Part model, mm, in its own coordinate system. A direction names the side the tool comes from. Coordinates: 2 decimals unless noted, no trailing zeros. Write each loop counter-clockwise with the first axis right and the second up, starting at its lowest first coordinate (ties: lowest second). Pieces come first, ordered by that corner, then holes. Notation, with made-up numbers: (-1.75, 51.25) - (29.25, 51.25) arc R18 cw to (29.25, 76.25) - close; hole circle Ø11 at (86, 62.25). An arc over 180 degrees is marked (long way). Use a Markdown table: item, result.
```python
from build123d import *

# Parameters (mm, degrees)
F3_DEPTH = 25.4
F4_R     = 3.175
F5_DEPTH = 18.3706396773


with BuildPart() as f1:
    # F0 (on Front) → F1 (revolve)
    with BuildSketch(Plane.XZ):
        with BuildLine():
            Line((6.35, 12.0196396773), (-120.65, 12.0196396773))
            Line((-120.65, 12.0196396773), (-120.65, 10.49467489))
            ThreePointArc((-120.65, 10.49467489), (-116.3146984161, 6.0237057619), (-114.733757664, 0))
            Line((-114.733757664, 0), (6.35, 0))
            Line((6.35, 0), (6.35, 12.0196396773))
        make_face()
    revolve(axis=Axis((-54.191878832, 0, 0), (-1, 0, 0)))

    # F2 (on face) → F3 (cut)
    with BuildSketch(Plane.YZ.offset(6.35)):
        with BuildLine():
            Line((-6.35, -10.2053533977), (-6.35, 10.2053533977))
            ThreePointArc((-6.35, 10.2053533977), (-12.0196396773, 0), (-6.35, -10.2053533977))
        make_face()
        with BuildLine():
            ThreePointArc((12.0196396773, 0), (10.5070559607, 5.8372521798), (6.35, 10.2053533977))
            Line((6.35, 10.2053533977), (6.35, -10.2053533977))
            ThreePointArc((6.35, -10.2053533977), (10.5070559607, -5.8372521798), (12.0196396773, 0))
        make_face()
    extrude(amount=-F3_DEPTH, mode=Mode.SUBTRACT)

    # F4 (on face) → F5 (cut, through all)
    with BuildSketch(Plane.XZ.offset(6.35)):
        Circle(F4_R)
    extrude(amount=-F5_DEPTH, mode=Mode.SUBTRACT)


solid = f1.part
```
Item 1: Band-saw the part on C-C, the plane y = 0. Give the cut face in (x, z) (3 decimals), then the cut area to 3 significant figures.
From the geometry:
| item | result |
|---|---|
| outline | (-120.65, -12.02) - (6.35, -12.02) - (6.35, 12.02) - (-120.65, 12.02) - (-120.65, 10.495) arc R12.266 cw to (-120.65, -10.495) - close; hole circle Ø6.35 at (0, 0) |
| area | 2,930 mm^2 |
Item 2: Which spindle directions (+Z, -Z, +X, -X, +Y, -Y) get a long thin tool onto all of the face, cutting with end or side? Do faces 1 (the face through (-19.05, -9, 0)), 2 (the face through (-6, 6.35, 0)), 3 (the face through (-72.15, 3.61, 11.465)). Say none if no direction does.
From the geometry:
| item | result |
|---|---|
| face 1 | +Z, -Z, +X, -Y |
| face 2 | +Z, -Z, +X, +Y |
| face 3 | +X, -X |
Item 3: Band-saw the part on A-A, the plane x = 0. Give the cut face in (y, z) (3 decimals).
From the geometry:
| item | result |
|---|---|
| outline | (-6.35, -10.205) arc R12.02 ccw to (6.35, -10.205) - (6.35, -3.175) - (-6.35, -3.175) - close; (-6.35, 3.175) - (6.35, 3.175) - (6.35, 10.205) arc R12.02 ccw to (-6.35, 10.205) - close |
Item 4: Band-saw the part on D-D, the plane x = -17. Give the cut face in (y, z), then the cut area to 3 significant figures.
From the geometry:
| item | result |
|---|---|
| outline | (-6.35, -10.21) arc R12.02 ccw to (6.35, -10.21) - (6.35, 10.21) arc R12.02 ccw to (-6.35, 10.21) - close |
| area | 290 mm^2 |
Item 5: Drop flat-ended pins along their axis: P1, Ø3, axis at y = -10.5, z = 3.5, coming from the +X side; P2, Ø10, axis at x = -12, z = -1, coming from the +Y side; P3, Ø3, axis at x = -38.5, z = 7.5, coming from the -Y side (3 decimals). Give the stop position or say it passes through.
From the geometry:
| item | result |
|---|---|
| P1 | x = -19.05 |
| P2 | y = 6.35 |
| P3 | y = -10.415 |
Item 6: Drill centre lines: probe 1 along Z at (x, y) = (0, 0.25) (3 decimals); probe 2 along Y at (x, z) = (-1, -9); probe 3 along Z at (x, y) = (0, 2.25) (3 decimals). Where is each one in solid material? Low to high.
From the geometry:
| item | result |
|---|---|
| probe 1 | -12.017 to -3.175, 3.175 to 12.017 |
| probe 2 | -6.35 to 6.35 |
| probe 3 | -11.807 to -3.175, 3.175 to 11.807 |
Item 7: Band-saw the part on B-B, the plane z = 0. Give the cut face in (x, y) (3 decimals).
From the geometry:
| item | result |
|---|---|
| outline | (-120.65, -12.02) - (-19.05, -12.02) - (-19.05, -6.35) - (-3.175, -6.35) - (-3.175, 6.35) - (-19.05, 6.35) - (-19.05, 12.02) - (-120.65, 12.02) - (-120.65, 10.495) arc R12.266 cw to (-120.65, -10.495) - close; (3.175, -6.35) - (6.35, -6.35) - (6.35, 6.35) - (3.175, 6.35) - close |
Item 8: Two-plate mould, pull along X, no slides. Class faces 4 (the face through (-120.65, -11, 0)), 5 (the face through (-0.69, -0.09, -3.1)), 6 (the face through (-6, -6.35, 0)), 7 (the face through (-19.05, 9, 0)): pulls with the +X half, pulls with the -X half, needs draft (parallel to the pull), parting line crosses it, or undercut.
From the geometry:
| item | result |
|---|---|
| face 4 | pulls with the -X half |
| face 5 | undercut |
| face 6 | needs draft |
| face 7 | pulls with the +X half |
